```python
from build123d import *

# Parameters (mm, degrees)
SKETCH1_W           = 288
SKETCH1_H           = 95
BOSS_EXTRUDE1_DEPTH = 3
SKETCH2_W           = 248
SKETCH2_H           = 75
BOSS_EXTRUDE2_DEPTH = 6
FILLET1_R           = 10
FILLET2_R           = 5


with BuildPart() as part:
    # Sketch1 → Boss-Extrude1 (new body)
    with BuildSketch(Plane(origin=(0, 0, 0), x_dir=(1, 0, 0), z_dir=(0, 1, 0))):
        with Locations((92.582008252, -21.664979636)):
            Rectangle(SKETCH1_W, SKETCH1_H)
    extrude(amount=BOSS_EXTRUDE1_DEPTH)

    # Sketch2 → Boss-Extrude2 (add)
    with BuildSketch(Plane.XZ):
        with Locations((92.582008252, 11.664979636)):
            Rectangle(SKETCH2_W, SKETCH2_H)
    extrude(amount=BOSS_EXTRUDE2_DEPTH)

    # Fillet1
    fillet1_edges = [part.edges().sort_by_distance(p)[0] for p in [
        (236.582008252, 1.5, -25.835020364),
        (-51.417991748, 1.5, -25.835020364),
        (236.582008252, 1.5, 69.164979636),
        (-51.417991748, 1.5, 69.164979636),
    ]]
    fillet(fillet1_edges, radius=FILLET1_R)

    # Fillet2
    fillet2_edges = [part.edges().sort_by_distance(p)[0] for p in [
        (-31.417991748, -3, 49.164979636),
        (-31.417991748, -3, -25.835020364),
        (216.582008252, -3, -25.835020364),
        (216.582008252, -3, 49.164979636),
    ]]
    fillet(fillet2_edges, radius=FILLET2_R)


solid = part.part
```
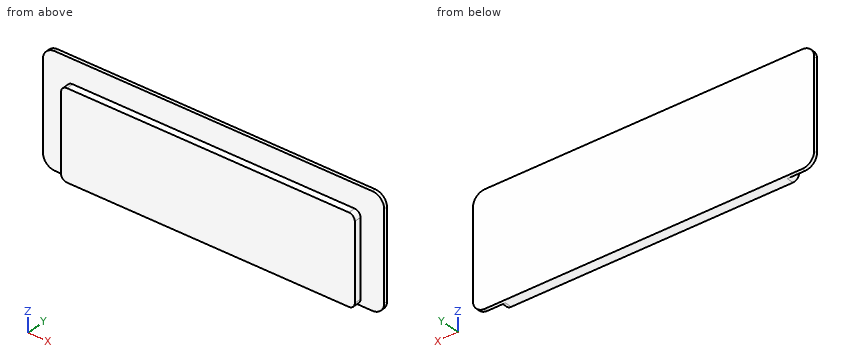
Geometry check sheet. Reference: the model listing, model coordinates, mm. Coordinates: 2 decimals unless noted, no trailing zeros. Order: outer loops, then holes, each group sorted by start corner. A loop starts at its lowest first (then second) coordinate and runs counter-clockwise, first axis right, second up. Notation, with made-up numbers: M 87.25,76.25 L 123.25,76.25 A28 ccw 123.25,114.25 Z; hole C -24.75,36.5 d7. An arc over 180 degrees is marked long. Answer as a JSON object with one key per item and string values.
Q1. Scan lines: line 1 (Y direction, x = 126, z = 65.5); line 2 (Z direction, x = 142, y = -3); line 3 (X direction, y = -1, z = 11). Record each from-to range of solid material in increasing order.
Results are:
{"line 1": "y = 0 to 3", "line 2": "z = -25.84 to 49.16", "line 3": "x = -31.42 to 216.58"}
Q2. Cross-section at A-A on y = -3.25. Record the cut outline in (x, z), and give its area (3 significant figures).
Results are:
{"outline": "M -31.42,-20.84 A5 ccw -26.42,-25.84 L 211.58,-25.84 A5 ccw 216.58,-20.84 L 216.58,44.16 A5 ccw 211.58,49.16 L -26.42,49.16 A5 ccw -31.42,44.16 Z", "area": "18,600 mm²"}
Q3. Cross-section at B-B on z = 7. Record the cut outline in (x, y), and give its area (3 significant figures).
Results are:
{"outline": "M -51.42,0 L -31.42,0 L -31.42,-6 L 216.58,-6 L 216.58,0 L 236.58,0 L 236.58,3 L -51.42,3 Z", "area": "2,350 mm²"}
Q4. Cross-section at C-C on x = 95.5. Record the cut outline in (y, z).
Results are:
{"outline": "M -6,-25.84 L 3,-25.84 L 3,69.16 L 0,69.16 L 0,49.16 L -6,49.16 Z"}
Q5. Depth check by flat-ended pin: pin 1 Ø1.5 at (y, z) = (-4, -3.5) entering from -X; pin 2 Ø5 at (y, z) = (-2, 24.5) entering from +X; pin 3 Ø1.8 at (x, y) = (87, -1.5) entering from +Z (3 decimals). Enter the tip coordinate at first touch or a pass-through.
Results are:
{"pin 1": "stops at x = -31.42", "pin 2": "stops at x = 236.58", "pin 3": "stops at z = 49.165"}
